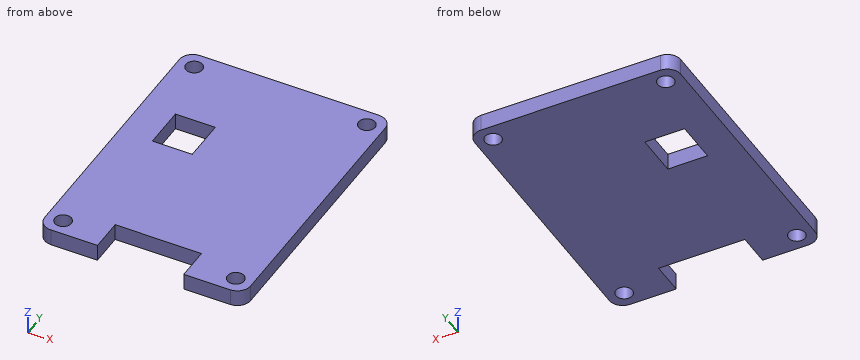
```python
from build123d import *

# Parameters (mm, degrees)
F0_R     = 1.25
F1_DEPTH = 2.5
F2_R     = 2


with BuildPart() as f1:
    # F0 (on Top) → F1 (new body)
    with BuildSketch(Plane.XY):
        Polygon((10.5, 16), (10.5, -16), (6.5, -16), (6.5, -21), (15.5, -21), (15.5, 21), (-15.5, 21), (-15.5, -21), (-6.5, -21), (-6.5, -16), (-10.5, -16), (-10.5, 2), (-10.5, 8.5), (-10.5, 16), align=None)
        with Locations((-13, -18.5)):
            Circle(F0_R, mode=Mode.SUBTRACT)
        with Locations((13, -18.5)):
            Circle(F0_R, mode=Mode.SUBTRACT)
        with Locations((-13, 18.5)):
            Circle(F0_R, mode=Mode.SUBTRACT)
        with Locations((13, 18.5)):
            Circle(F0_R, mode=Mode.SUBTRACT)
        Polygon((6.5, -16), (10.5, -16), (10.5, 16), (-10.5, 16), (-10.5, 8.5), (-4.5, 8.5), (-4.5, 2), (-10.5, 2), (-10.5, -16), (-6.5, -16), align=None)
    extrude(amount=F1_DEPTH)

    # F2
    f2_edges = [f1.edges().sort_by_distance(p)[0] for p in [
        (-15.5, 21, 1.25),
        (15.5, 21, 1.25),
        (15.5, -21, 1.25),
        (-15.5, -21, 1.25),
    ]]
    fillet(f2_edges, radius=F2_R)


solid = f1.part
```
Part model, mm, in its own coordinate system. Coordinates: 2 decimals unless noted, no trailing zeros. Order: outer loops, then holes, each group sorted by start corner. A loop starts at its lowest first (then second) coordinate and runs counter-clockwise, first axis right, second up. Notation, with made-up numbers: (-1, 65) - (40, 65) arc R19 cw to (40, 81) - close; hole circle Ø8 at (-28, 34.5). An arc over 180 degrees is marked (long way). Return JSON: item names as keys, results as strings. Group by question number.
Item 1: Cut at B-B (z = 1.5). List the corners of the cut face in (x, y), plus the area to 3 significant figures.
Item 2: Cut at A-A (y = 18.5). List the corners of the cut face in (x, z).
Item 3: Drill centre lines: probe 1 along Y at (x, z) = (13, 1.3); probe 2 along Y at (x, z) = (12, 1.25); probe 3 along Y at (x, z) = (-7, 0.65). Where is each one in solid material? Low to high. Write a range as from..to.
Item 4: Cut at C-C (x = -9). List the corners of the cut face in (y, z), plus the area to 4 significant figures.
Item 5: Pin check, flat tips, straight feed: pin 1 (0.8 mm diameter, centred on x = -2.5, z = 2, fed in from -Y); pin 2 (2 mm diameter, centred on x = 1, y = -4.5, fed in from -Z); pin 3 (2 mm diameter, centred on x = 13, y = -18.5, fed in from +Z) (3 decimals). Stop position of each tip, or through.
Item 6: Cut at D-D (y = -18.5). List the corners of the cut face in (x, z).
Check values:
{
 "1": {"outline": "(-15.5, -19) arc R2 ccw to (-13.5, -21) - (-6.5, -21) - (-6.5, -16) - (6.5, -16) - (6.5, -21) - (13.5, -21) arc R2 ccw to (15.5, -19) - (15.5, 19) arc R2 ccw to (13.5, 21) - (-13.5, 21) arc R2 ccw to (-15.5, 19) - close; hole circle Ø2.5 at (-13, -18.5); hole circle Ø2.5 at (-13, 18.5); hole (-10.5, 2) - (-4.5, 2) - (-4.5, 8.5) - (-10.5, 8.5) - close; hole circle Ø2.5 at (13, -18.5); hole circle Ø2.5 at (13, 18.5)", "area": "1,170 mm2"},
 "2": {"outline": "(-15.5, 0) - (-14.25, 0) - (-14.25, 2.5) - (-15.5, 2.5) - close; (-11.75, 0) - (11.75, 0) - (11.75, 2.5) - (-11.75, 2.5) - close; (14.25, 0) - (15.5, 0) - (15.5, 2.5) - (14.25, 2.5) - close"},
 "3": {"probe 1": "y = -21..-19.75, -17.25..17.25, 19.75..21", "probe 2": "y = -21..-19.25, -17.75..17.75, 19.25..21", "probe 3": "y = -21..2, 8.5..21"},
 "4": {"outline": "(-21, 0) - (2, 0) - (2, 2.5) - (-21, 2.5) - close; (8.5, 0) - (21, 0) - (21, 2.5) - (8.5, 2.5) - close", "area": "88.75 mm2"},
 "5": {"pin 1": "stops at y = -16", "pin 2": "stops at z = 0", "pin 3": "passes through"},
 "6": {"outline": "(-15.5, 0) - (-14.25, 0) - (-14.25, 2.5) - (-15.5, 2.5) - close; (-11.75, 0) - (-6.5, 0) - (-6.5, 2.5) - (-11.75, 2.5) - close; (6.5, 0) - (11.75, 0) - (11.75, 2.5) - (6.5, 2.5) - close; (14.25, 0) - (15.5, 0) - (15.5, 2.5) - (14.25, 2.5) - close"}
}
